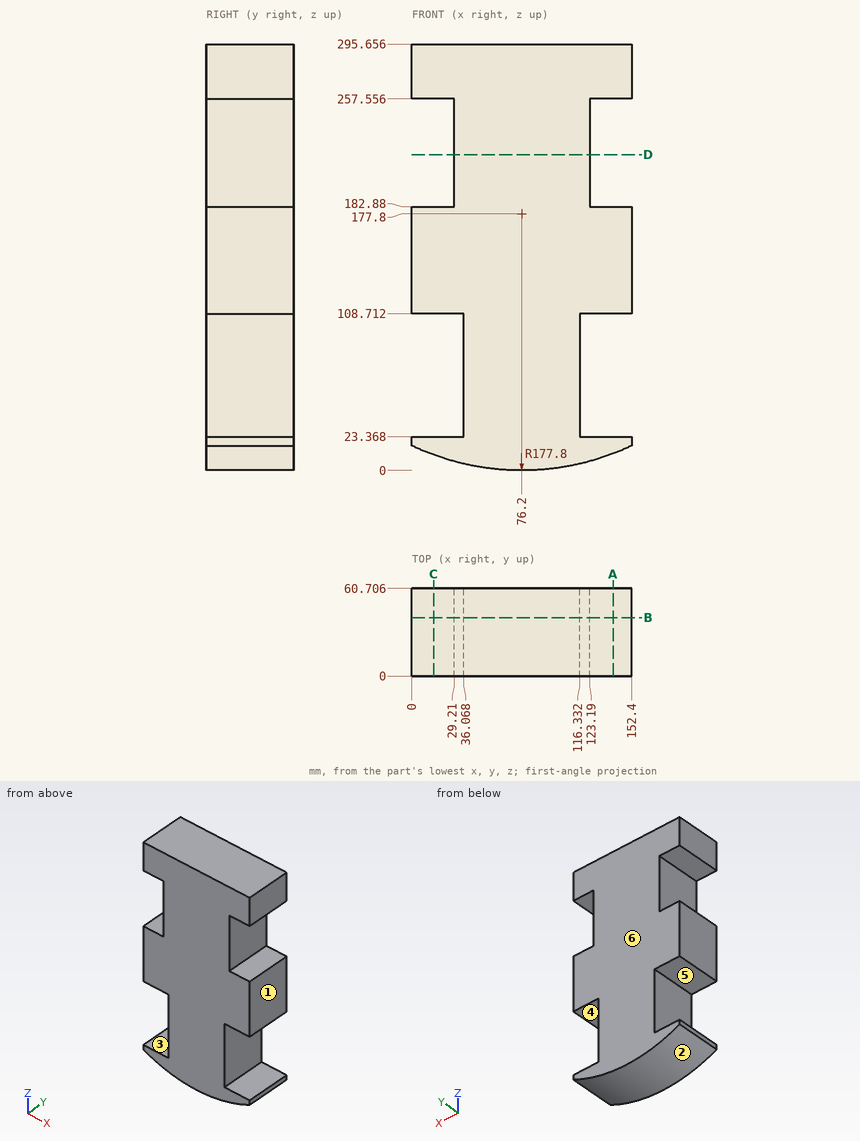
Could you check a few things on this drawing? It's one solid part, dimensions in mm from its lowest x, y, z. A direction names the side the tool comes from. Give positions to 0.01 mm unless a question says otherwise; leave off trailing zeros. Order: outer loops, then holes, each group sorted by start corner. A loop starts at its lowest first (then second) coordinate and runs counter-clockwise, first axis right, second up. Notation, with made-up numbers: (-17, 77) -> (16, 77) arc R24 cw to (16, 103) -> close; hole circle Ø5 at (-11.75, 40.5). An arc over 180 degrees is marked (long way). Use CSV: the item, a comma, the result in double quotes. Start each with the question number.
Item 1: Suppose I cut it at A-A (x = 139.5). List the corners of the cut face in (y, z) for me.
Item 2: On a 3-axis mill with a long thin cutter (end or side, diameter ignored), from which of +Z, -Z, +X, -X, +Y, -Y can I reach the whole of each face in a straight line? I mean the marked faces 4, 5 and 6. Say none if no direction works.
Item 3: Suppose I cut it at C-C (x = 15). List the corners of the cut face in (y, z) for me.
Item 4: I'm going to push flat-ended pins straight in: P1, Ø5, axis at y = 36, z = 61, coming from the -X side; P2, Ø3, axis at y = 13.5, z = 55.5, coming from the +X side; P3, Ø9, axis at x = 144.5, y = 32.5, coming from the -Z side. Where does each tip first touch, or does it pass through?
Item 5: If I drill on probe 1 along Z at (x, y) = (136, 37); probe 2 along Z at (x, y) = (22.5, 52.5); probe 3 along Z at (x, y) = (72.5, 24.5), over which ranges is the centre line in solid material (lowest first)? Write a range as [from, to].
Item 6: Suppose I cut it at B-B (y = 40.5). List the corners of the cut face in (x, z) for me.
Item 7: Thinking about a two-plate mould opening in Z: for the marked faces 1, 2 and 3, which applies, pulls with the +Z half, pulls with the -Z half, needs draft (parallel to the pull), parting line crosses it, or undercut?
Item 8: Suppose I cut it at D-D (z = 219). List the corners of the cut face in (x, y) for me.
Answer block:
1,outline,"(0, 11.65) -> (60.71, 11.65) -> (60.71, 23.37) -> (0, 23.37) -> close; (0, 108.71) -> (60.71, 108.71) -> (60.71, 182.88) -> (0, 182.88) -> close; (0, 257.56) -> (60.71, 257.56) -> (60.71, 295.66) -> (0, 295.66) -> close"
2,face 4,"+X, +Y, -Y"
2,face 5,"-X, +Y, -Y"
2,face 6,"+Z, -Z, +X, -X, +Y"
3,outline,"(0, 10.86) -> (60.71, 10.86) -> (60.71, 23.37) -> (0, 23.37) -> close; (0, 108.71) -> (60.71, 108.71) -> (60.71, 182.88) -> (0, 182.88) -> close; (0, 257.56) -> (60.71, 257.56) -> (60.71, 295.66) -> (0, 295.66) -> close"
4,P1,"stops at x = 36.07"
4,P2,"stops at x = 116.33"
4,P3,"stops at z = 11.84"
5,probe 1,"z = [10.36, 23.37], [108.71, 182.88], [257.56, 295.66]"
5,probe 2,"z = [8.3, 23.37], [108.71, 182.88], [257.56, 295.66]"
5,probe 3,"z = [0.04, 295.66]"
6,outline,"(0, 17.16) arc R177.8 ccw to (152.4, 17.16) -> (152.4, 23.37) -> (116.33, 23.37) -> (116.33, 108.71) -> (152.4, 108.71) -> (152.4, 182.88) -> (123.19, 182.88) -> (123.19, 257.56) -> (152.4, 257.56) -> (152.4, 295.66) -> (0, 295.66) -> (0, 257.56) -> (29.21, 257.56) -> (29.21, 182.88) -> (0, 182.88) -> (0, 108.71) -> (36.07, 108.71) -> (36.07, 23.37) -> (0, 23.37) -> close"
7,face 1,"needs draft"
7,face 2,"pulls with the -Z half"
7,face 3,"undercut"
8,outline,"(29.21, 0) -> (123.19, 0) -> (123.19, 60.71) -> (29.21, 60.71) -> close"
